```python
from build123d import *

# Parameters (mm, degrees)
SKETCH1_R           = 12
BOSS_EXTRUDE1_DEPTH = 8
CHAMFER1_SIZE       = 1
SKETCH2_R           = 8
BOSS_EXTRUDE2_DEPTH = 8


with BuildPart() as part:
    # Sketch1 → Boss-Extrude1 (new body)
    with BuildSketch(Plane.XY):
        Circle(SKETCH1_R)
    extrude(amount=BOSS_EXTRUDE1_DEPTH)

    # Chamfer1
    chamfer1_edges = [part.edges().sort_by_distance(p)[0] for p in [
        (-12, 0, 8),
    ]]
    chamfer(chamfer1_edges, length=CHAMFER1_SIZE)

    # Sketch2 → Boss-Extrude2 (add)
    with BuildSketch(Plane(origin=(0, 0, 0), x_dir=(-1, 0, 0), z_dir=(0, 0, -1))):
        Circle(SKETCH2_R)
    extrude(amount=BOSS_EXTRUDE2_DEPTH)


solid = part.part
```
Verification items for the finished model (mm, model axes). A direction names the side the tool comes from. Give positions to 0.01 mm unless a question says otherwise; leave off trailing zeros. Order: outer loops, then holes, each group sorted by start corner. A loop starts at its lowest first (then second) coordinate and runs counter-clockwise, first axis right, second up. Notation, with made-up numbers: (-31.5, -33.5) -> (6.5, -33.5) arc R27 cw to (6.5, -5.5) -> close; hole circle Ø6 at (40, 78). An arc over 180 degrees is marked (long way). One line per item, written item: value.
(1) Gauge pin test, flat ends, axial feed: pin 1 (1 mm diameter, centred on x = -3, z = -3.5, fed in from -Y); pin 2 (6 mm diameter, centred on x = 7, z = -4, fed in from -Y); pin 3 (1 mm diameter, centred on y = 7, z = 1.5, fed in from +X). Record the tip position at first contact, or that the pin passes through.
Final values:
pin 1: y = -7.6
pin 2: y = -6.93
pin 3: x = 10.09
(2) Sectioned sample at D-D on z = -6.5. Record the cut outline in (x, y).
Final values:
outline: circle Ø16 at (0, 0)
(3) Sectioned sample at C-C on z = 2.5. Record the cut outline in (x, y), then the cut area to 3 significant figures.
Final values:
outline: circle Ø24 at (0, 0)
area: 452 mm^2
(4) Tool access check on faces 1 (the face through (1.73, -7.81, -3.94)), 2 (the face through (0, 0, -8)). Record the directions out of +Z, -Z, +X, -X, +Y, -Y that give a thin tool (end or side, any length) a straight path to the whole face; none if there is none.
Final values:
face 1: -Z
face 2: -Z, +X, -X, +Y, -Y
(5) Sectioned sample at A-A on y = 0. Record the cut outline in (x, z).
Final values:
outline: (-12, 0) -> (-8, 0) -> (-8, -8) -> (8, -8) -> (8, 0) -> (12, 0) -> (12, 7) -> (11, 8) -> (-11, 8) -> (-12, 7) -> close
(6) Scan lines: line 1 along Z through (x, y) = (-9.75, 0.5); line 2 along Y through (x, z) = (-4.75, -2.25); line 3 along Y through (x, z) = (-9.25, 6.5). Record each from-to range of solid material in increasing order. Write a range as [from, to].
Final values:
line 1: [0, 8]
line 2: [-6.44, 6.44]
line 3: [-7.64, 7.64]
